Autodesk Inventor part; units mm, degrees
ref_plane "Work Plane1" through (0, 4, 0) normal (0, 1, 0) x (-1, 0, 0)
ref_plane "YZ Plane" through (0, 0, 0) normal (1, 0, 0) x (0, 1, 0)
ref_plane "XY Plane" through (0, 0, 0) normal (0, 0, 1) x (1, 0, 0)
sketch "Sketch1" plane through (0, 0, 0) normal (0, 0, 1) x (1, 0, 0)
  circle A0 centre (0, 0) radius 4
  dimension "d0" = 8
extrude "Extrusion1" add sketch "Sketch1" against normal blind 260
ref_plane "Work Plane1" through (0, 4, 0) normal (0, 1, 0) x (-1, 0, 0)
sketch "Sketch2" plane through (0, 4, 0) normal (0, 1, 0) x (-1, 0, 0)
  line L0 (-4, -260) -> (4, -260) construction
  line L1 (4, 0) -> (-4, 0) construction
  point P0 (0, 0)
  point P1 (0, -5)
  dimension "d11" = 5
hole "Hole1" at (0, 4, -5) direction (0, -1, 0) diameter 3.688 end through all
sketch "Sketch3" plane through (0, 4, 0) normal (0, 1, 0) x (-1, 0, 0)
  line L0 (-4, -260) -> (4, -260) construction
  line L1 (0, -260) -> (0, -249.076) construction
  point P0 (0, 0)
  dimension "d12" = 10.924
hole "Hole2" at (0, 4, -249.076) direction (0, -1, 0) diameter 3.688 end through all
sketch "Sketch4" plane through (0, 0, 0) normal (0, 0, 1) x (1, 0, 0)
  circle A0 centre (0, 0) radius 2.5
  dimension "d20" = 5
extrude "Extrusion2" cut sketch "Sketch4" against normal blind 13.274
properties part number "driveshaft" material "Steel, Mild"
Here's how the part is built. I have some questions about the finished solid (model axes, mm). A direction names the side the tool comes from. Coordinates: 2 decimals unless noted, no trailing zeros. Order: outer loops, then holes, each group sorted by start corner. A loop starts at its lowest first (then second) coordinate and runs counter-clockwise, first axis right, second up. Notation, with made-up numbers: M 47.5,13.5 L 63.5,13.5 A20 ccw 63.5,50.5 Z; hole C -25.75,-9.75 d1. An arc over 180 degrees is marked long. Answer as a JSON object with one key per item and string values. Group by question number.
(1) For pin 1 (1 mm diameter, centred on x = -1, z = -167.5, fed in from -Y); pin 2 (3 mm diameter, centred on x = 2.5, z = -174.5, fed in from -Y); pin 3 (4 mm diameter, centred on x = 0, y = 0, fed in from +Z), each with a flat end and sliding along its axis, tell me the tip position at first contact or that it passes through.
(2) Suppose I cut it at B-B, the plane y = 0. Please give me the cut outline in (x, z).
(3) Suppose I cut it at A-A, the plane x = 0. Please give me the cut outline in (y, z).
(4) Which directions (+Z, -Z, +X, -X, +Y, -Y) give clear straight access to the entire face, cutting with the end or side of a thin tool? Please do faces 4 (the face through (2.385, 0.751, -6.544)), 5 (the face through (0, 0, -260)).
(5) Suppose I cut it at C-C, the plane z = -228. Please give me the cut outline in (x, y).
(6) I need wall thicknesses on probe 1 along Z at (x, y) = (0, -3.5); probe 2 along Z at (x, y) = (0, -0.75); probe 3 along Z at (x, y) = (1.25, -3). Which ranges of each line are inside material? Lowest first, please.
(7) If we mould it in two halves opening along X, with no side actions, what happens to faces 1 (the face through (-0.867, -3.905, -128.18)), 2 (the face through (0, 0, -13.274)), 3 (the face through (2, 2, 0))? For each: released by +X, released by -X, zero draft, split by the parting line, or undercut.
Values found:
{
 "1": {"pin 1": "stops at y = -3.97", "pin 2": "stops at y = -3.87", "pin 3": "stops at z = -13.27"},
 "2": {"outline": "M -4,-260 L 4,-260 L 4,0 L 2.5,0 L 2.5,-13.27 L -2.5,-13.27 L -2.5,0 L -4,0 Z; hole C 0,-249.08 d3.69"},
 "3": {"outline": "M -4,-260 L 4,-260 L 4,-250.92 L -4,-250.92 Z; M -4,-247.23 L 4,-247.23 L 4,-6.84 L 2.5,-6.84 L 2.5,-13.27 L -2.5,-13.27 L -2.5,-6.84 L -4,-6.84 Z; M -4,-3.16 L -2.5,-3.16 L -2.5,0 L -4,0 Z; M 2.5,-3.16 L 4,-3.16 L 4,0 L 2.5,0 Z"},
 "4": {"face 4": "+Z", "face 5": "-Z, +X, -X, +Y, -Y"},
 "5": {"outline": "C 0,0 d8"},
 "6": {"probe 1": "z = -260 to -250.92, -247.23 to -6.84, -3.16 to 0", "probe 2": "z = -260 to -250.92, -247.23 to -13.27", "probe 3": "z = -260 to -250.43, -247.72 to -6.36, -3.64 to 0"},
 "7": {"face 1": "split by the parting line", "face 2": "undercut", "face 3": "zero draft"}
}
